Work out the finished part from the listing and answer in its coordinate system (mm). Face numbers are marked on the shaded views. Coordinates: 2 decimals unless noted, no trailing zeros. Order: outer loops, then holes, each group sorted by start corner. A loop starts at its lowest first (then second) coordinate and runs counter-clockwise, first axis right, second up. Notation, with made-up numbers: (-33.5, -22.5) -> (-0.5, -22.5) arc R17 ccw to (-0.5, -4.5) -> close; hole circle Ø7 at (33.5, -4). An arc over 180 degrees is marked (long way). Write item = value, one per line. Start each with the question number.
Q1. The part is cut by section A-A, the plane x = 0. Determine the outline of the cut face in (y, z).
Q2. For a pull along Z with two mould halves and no side action, classify the marked faces 1, 2 and 3 as +Z half, -Z half, draft (parallel to the pull), parting line (faces both ways), or undercut.
Q3. Flat-ended cylindrical pins translate along their axes: pin 1 (1.5 mm diameter, centred on x = 44.5, y = -33.5, fed in from -Z); pin 2 (1.5 mm diameter, centred on y = -53, z = 10.5, fed in from +X); pin 3 (10 mm diameter, centred on y = -31.5, z = -17.5, fed in from -X). Find the tip coordinate at first contact, or state that the pin passes through.
Q4. The part is cut by section C-C, the plane y = -42. Determine the outline of the cut face in (x, z), plus the area to 3 significant figures.
Q5. Straight lines are drawn through the part: L1, parallel to Z at x = 0, y = -18; L2, parallel to X at y = -40.5, z = 11; L3, parallel to Z at x = -9.5, y = -26. For each, find the intervals that lie inside material, in ascending order. Write a range as from..to.
Q6. The part is cut by section B-B, the plane z = 16. Determine the outline of the cut face in (x, y), plus the area to 3 significant figures.
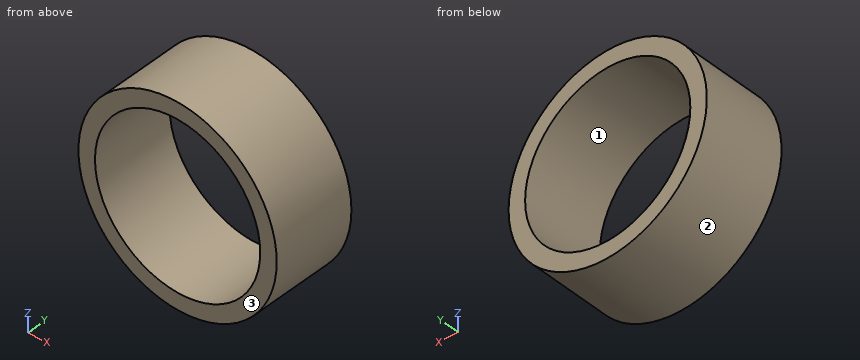
```python
from build123d import *

# Parameters (mm, degrees)
F0_R     = 72.2228243582
F1_DEPTH = 10
F2_R     = 72.2228243582
F3_DEPTH = 25.4
F5_R     = 13.3709609509
F6_DEPTH = 226
F4_R     = 60.1818073618
F7_DEPTH = 139.5800691098
F8_DEPTH = 25


# Not quite as in the source:
# - an extrude ends at something that could not be found from the text; its depth is read off the source's solid


with BuildPart() as f1:
    # F0 (on Front) → F1 (new body)
    with BuildSketch(Plane.XZ):
        Circle(F0_R)
    extrude(amount=F1_DEPTH)

    # F2 (on face) → F3 (join)
    with BuildSketch(Plane.XZ.offset(10)):
        Circle(F2_R)
    extrude(amount=F3_DEPTH)

    # F5 (on Front) → F6 (cut, through all)
    with BuildSketch(Plane.XZ):
        with Locations((0, 13.3709609509)):
            Circle(F5_R)
    extrude(amount=-F6_DEPTH, mode=Mode.SUBTRACT)

    # F4 (on face) → F7 (cut)
    with BuildSketch(Plane(origin=(0, 0, 0), x_dir=(-1, 0, 0), z_dir=(0, 1, 0))):
        Circle(F4_R)
    extrude(amount=-F7_DEPTH, mode=Mode.SUBTRACT)

    # F8 (add): a face of the model
    f8_faces = [f1.faces().sort_by_distance(p)[0] for p in [
        (-70.1800544038, -35.4, 0),
    ]]
    extrude(f8_faces, amount=F8_DEPTH)


solid = f1.part
```
Model answer:
q1.outline = (-60.4, -72.22) -> (0, -72.22) -> (0, -60.18) -> (-60.4, -60.18) -> close; (-60.4, 60.18) -> (0, 60.18) -> (0, 72.22) -> (-60.4, 72.22) -> close
q2.face_1 = undercut
q2.face_2 = parting line
q2.face_3 = draft
q3.pin_1 = -57.46
q3.pin_2 = 71.56
q3.pin_3 = -71.13
q4.outline = circle Ø144.45 at (0, 0); hole circle Ø120.36 at (0, 0)
q4.area = 5,010 mm2
q5.L1 = -72.22..-60.18, 60.18..72.22
q5.L2 = -71.38..-59.17, 59.17..71.38
q5.L3 = -71.6..-59.43, 59.43..71.6
q6.outline = (-70.43, -60.4) -> (-58.02, -60.4) -> (-58.02, 0) -> (-70.43, 0) -> close; (58.02, -60.4) -> (70.43, -60.4) -> (70.43, 0) -> (58.02, 0) -> close
q6.area = 1,500 mm2
